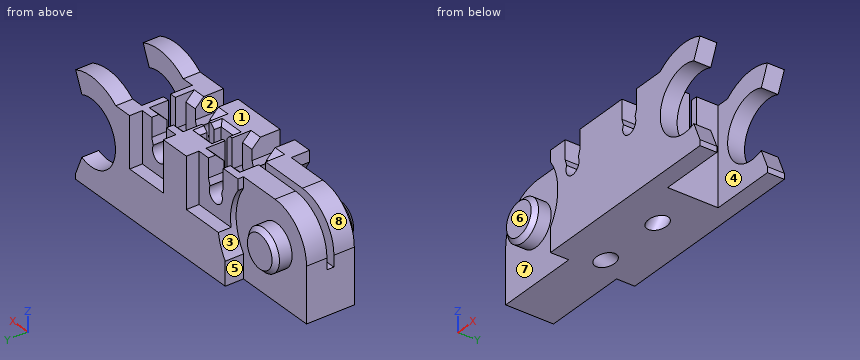
```python
from build123d import *

# Parameters (mm, degrees)
BOSS_EXTRUDE7_DEPTH      = 20
SKETCH2_R                = 4.9175
BOSS_EXTRUDE2_DEPTH      = 4
CUT_EXTRUDE1_REACH       = 70.602
SKETCH3_R                = 7.665
SKETCH4_W                = 4
SKETCH4_H                = 5
CUT_EXTRUDE2_DEPTH       = 10
BOSS_EXTRUDE4_DEPTH      = 4
BOSS_EXTRUDE5_START      = -4
BOSS_EXTRUDE5_DEPTH      = 4
SKETCH25_R               = 12.83
SKETCH25_R_2             = 4.9175
CUT_EXTRUDE9_DEPTH       = 4.33
CUT_EXTRUDE10_START      = -4.33
CUT_EXTRUDE10_DEPTH      = 4.33
CUT_EXTRUDE5_DEPTH       = 70.42587576
SKETCH17_W               = 10.66
SKETCH17_H               = 6.66
CUT_EXTRUDE6_DEPTH       = 7
SKETCH18_W               = 3.2475
SKETCH18_H               = 6.66
SKETCH19_W               = 3.2475
SKETCH19_H               = 6.66
SKETCH20_W               = 51.84
SKETCH20_H               = 1.66
CUT_EXTRUDE7_DEPTH       = 12.66
CHAMFER2_SIZE            = 1
CHAMFER3_SIZE            = 1
CHAMFER4_SIZE            = 2
FILLET1_R                = 10
BOSS_EXTRUDE13_REACH     = 70.3
SKETCH23_W               = 10.34
SKETCH23_H               = 1.66
BOSS_EXTRUDE14_DEPTH     = 0.360269713
SKETCH24_W               = 12.33
SKETCH24_H               = 12
SKETCH24_W_2             = 10.66
CUT_EXTRUDE8_DEPTH       = 3
CHAMFER5_SIZE            = 1
CUT_EXTRUDE11_DEPTH      = 14
CUT_EXTRUDE11_DEPTH_BACK = 14
SKETCH27_R               = 2.0825
SKETCH28_R               = 2.0825
CUT_EXTRUDE12_DEPTH      = 14


with BuildPart() as part:
    # Sketch16 → Boss-Extrude7 (new body)
    with BuildSketch(Plane.XY):
        Polygon((-42.5, -10), (0, -10), (3, -10), (3, -6), (0, -6), (-10.66, -6), (-10.66, 6), (0, 6), (3, 6), (3, 10), (0, 10), (-42.5, 10), (-42.5, 5.67), (-53, 5.67), (-62.5, 5.67), (-62.5, -5.67), (-53, -5.67), (-42.5, -5.67), align=None)
    extrude(amount=BOSS_EXTRUDE7_DEPTH)

    # Sketch2 → Boss-Extrude2 (add)
    with BuildSketch(Plane.XZ.offset(5.67)):
        with Locations(Location((-53, 10, 0), (0, 0, 180))):
            Circle(SKETCH2_R)
    boss_extrude2 = extrude(amount=BOSS_EXTRUDE2_DEPTH)

    # Cut-Extrude1: up to this face of the body (flat: up to its plane)
    cut_extrude1_end = Plane(part.part.faces().sort_by_distance((-19.75, 10, 10))[0])
    # Sketch3 → Cut-Extrude1 (cut, up to the picked face)
    with BuildSketch(Plane.XZ.offset(10), mode=Mode.PRIVATE) as cut_extrude1_sk1:
        with Locations((0, 10)):
            Circle(SKETCH3_R)
    cut_extrude1_tool1 = split(extrude(cut_extrude1_sk1.sketch, amount=-CUT_EXTRUDE1_REACH, mode=Mode.PRIVATE), bisect_by=cut_extrude1_end, keep=Keep.BOTH, mode=Mode.PRIVATE)
    add(cut_extrude1_tool1.solids().sort_by(Axis((0, -10, 10), (0, 1, 0)))[0], mode=Mode.SUBTRACT)

    # Mirror1: Boss-Extrude2 across plane
    add(boss_extrude2.mirror(Plane.ZX))

    # Sketch4 → Cut-Extrude2 (cut)
    with BuildSketch(Plane.XY.offset(20)):
        with Locations((-26.5, 0)):
            Rectangle(SKETCH4_W, SKETCH4_H)
    extrude(amount=-CUT_EXTRUDE2_DEPTH, mode=Mode.SUBTRACT)

    # Sketch10 → Boss-Extrude4 (add)
    with BuildSketch(Plane.XZ.offset(10)):
        with BuildLine():
            Line((3, 17.053525714), (4.956947162, 21.654651425))
            ThreePointArc((4.956947162, 21.654651425), (-12.665, 10), (4.956947162, -1.654651425))
            Line((4.956947162, -1.654651425), (3, 2.946474286))
            ThreePointArc((3, 2.946474286), (-7.665, 10), (3, 17.053525714))
        make_face()
    extrude(amount=-BOSS_EXTRUDE4_DEPTH)

    # Sketch11 → Boss-Extrude5 (add)
    with BuildSketch(Plane(origin=(0, 10, 0), x_dir=(1, 0, 0), z_dir=(0, 1, 0)).offset(BOSS_EXTRUDE5_START)):
        with BuildLine():
            Line((4.956947162, -21.654651425), (3, -17.053525714))
            ThreePointArc((3, -17.053525714), (-7.665, -10), (3, -2.946474286))
            Line((3, -2.946474286), (4.956947162, 1.654651425))
            ThreePointArc((4.956947162, 1.654651425), (-1.632617278, 2.559330628), (-7.771886837, 0))
            Line((-7.771886837, 0), (-10.66, 0))
            Line((-10.66, 0), (-10.66, -20))
            Line((-10.66, -20), (-7.771886837, -20))
            ThreePointArc((-7.771886837, -20), (-1.632617278, -22.559330628), (4.956947162, -21.654651425))
        make_face()
    extrude(amount=BOSS_EXTRUDE5_DEPTH)

    # Sketch25 → Cut-Extrude9 (cut)
    with BuildSketch(Plane.XZ.offset(10)):
        with Locations((-53, 10)):
            Circle(SKETCH25_R)
        with Locations(Location((-53, 10, 0), (0, 0, 180))):
            Circle(SKETCH25_R_2, mode=Mode.SUBTRACT)
    extrude(amount=-CUT_EXTRUDE9_DEPTH, mode=Mode.SUBTRACT)

    # Sketch26 → Cut-Extrude10 (cut)
    with BuildSketch(Plane(origin=(0, 10, 0), x_dir=(1, 0, 0), z_dir=(0, 1, 0)).offset(CUT_EXTRUDE10_START)):
        with BuildLine():
            Line((-42.5, -2.627151161), (-42.5, -17.372848839))
            ThreePointArc((-42.5, -17.372848839), (-40.17, -10), (-42.5, -2.627151161))
        make_face()
    extrude(amount=CUT_EXTRUDE10_DEPTH, mode=Mode.SUBTRACT)

    # Sketch13 → Cut-Extrude5 (cut, through all)
    with BuildSketch(Plane.XZ.offset(10)):
        with BuildLine():
            Line((-37.83, 15.484673169), (-37.83, 20))
            Line((-37.83, 20), (-33.17, 20))
            Line((-33.17, 20), (-33.17, 15.484673169))
            Line((-33.17, 15.484673169), (-33.665, 13.984673169))
            ThreePointArc((-33.665, 13.984673169), (-35.5, 10.9175), (-37.335, 13.984673169))
            Line((-37.335, 13.984673169), (-37.83, 15.484673169))
        make_face()
        with BuildLine():
            Line((-19.83, 15.484673169), (-19.83, 20))
            Line((-19.83, 20), (-15.17, 20))
            Line((-15.17, 20), (-15.17, 15.484673169))
            Line((-15.17, 15.484673169), (-15.665, 13.984673169))
            ThreePointArc((-15.665, 13.984673169), (-17.5, 10.9175), (-19.335, 13.984673169))
            Line((-19.335, 13.984673169), (-19.83, 15.484673169))
        make_face()
    extrude(amount=-CUT_EXTRUDE5_DEPTH, mode=Mode.SUBTRACT)

    # Sketch17 → Cut-Extrude6 (cut)
    with BuildSketch(Plane.XY.offset(20)):
        with Locations((-35.5, 0)):
            Rectangle(SKETCH17_W, SKETCH17_H)
        with Locations((-17.5, 0)):
            Rectangle(SKETCH17_W, SKETCH17_H)
    extrude(amount=-CUT_EXTRUDE6_DEPTH, mode=Mode.SUBTRACT)

    # Sketch18 → Cut-Revolve1 (revolve, cut)
    with BuildSketch(Plane.XY.offset(13)):
        with Locations((-39.20625, 0)):
            Rectangle(SKETCH18_W, SKETCH18_H)
    revolve(axis=Axis((-35.5, 10, 13), (0, -1, 0)), mode=Mode.SUBTRACT)

    # Sketch19 → Cut-Revolve2 (revolve, cut)
    with BuildSketch(Plane.XY.offset(13)):
        with Locations((-21.20625, 0)):
            Rectangle(SKETCH19_W, SKETCH19_H)
    revolve(axis=Axis((-17.5, 10, 13), (0, -1, 0)), mode=Mode.SUBTRACT)

    # Sketch20 → Cut-Extrude7 (cut)
    with BuildSketch(Plane.XY.offset(20)):
        with Locations((-36.58, 0)):
            Rectangle(SKETCH20_W, SKETCH20_H)
    extrude(amount=-CUT_EXTRUDE7_DEPTH, mode=Mode.SUBTRACT)

    # Chamfer2
    chamfer2_edges = [part.edges().sort_by_distance(p)[0] for p in [
        (-48.0825, -9.67, 10),
    ]]
    chamfer(chamfer2_edges, length=CHAMFER2_SIZE)

    # Chamfer3
    chamfer3_edges = [part.edges().sort_by_distance(p)[0] for p in [
        (-48.0825, 9.67, 10),
    ]]
    chamfer(chamfer3_edges, length=CHAMFER3_SIZE)

    # Chamfer4
    chamfer4_edges = [part.edges().sort_by_distance(p)[0] for p in [
        (-31.67, -3.33, 20),
        (-31.67, 3.33, 20),
        (-39.33, 3.33, 20),
        (-39.33, -3.33, 20),
        (-13.67, -3.33, 20),
        (-13.67, 3.33, 20),
        (-21.33, 3.33, 20),
        (-21.33, -3.33, 20),
    ]]
    chamfer(chamfer4_edges, length=CHAMFER4_SIZE)

    # Fillet1
    # the kernel refuses this fillet: 10 mm, written as the material it takes off along each edge
    with BuildSketch(Plane(origin=(-62.5, 30.67, 0), x_dir=(1, 0, 0), z_dir=(0, -1, 0))) as fillet1_piece_1:
        with BuildLine():
            CenterArc((FILLET1_R, FILLET1_R), FILLET1_R, 180, 90)
            Line((0, FILLET1_R), (0, 0))
            Line((0, 0), (FILLET1_R, 0))
        make_face()
    extrude(amount=61.34, mode=Mode.SUBTRACT)
    with BuildSketch(Plane(origin=(-62.5, 30.67, 20), x_dir=(1, 0, 0), z_dir=(0, -1, 0)), Plane(origin=(-62.5, 24.17, 20), x_dir=(1, 0, 0), z_dir=(0, -1, 0))) as fillet1_piece_2:
        with BuildLine():
            CenterArc((FILLET1_R, -FILLET1_R), FILLET1_R, 90, 90)
            Line((0, -FILLET1_R), (0, 0))
            Line((0, 0), (FILLET1_R, 0))
        make_face()
    extrude(amount=54.84, mode=Mode.SUBTRACT)

    # Sketch22 → Boss-Extrude13 (add, up to next)
    with BuildSketch(Plane(origin=(0, 0, -3), x_dir=(-1, 0, 0), z_dir=(0, 0, -1)), mode=Mode.PRIVATE) as boss_extrude13_sk1:
        Polygon((62.5, 5.67), (52.5, 5.67), (42.5, 5.67), (42.5, 10), (7.771886837, 10), (-4.956947162, 10), (-4.956947162, 6), (7.771886837, 6), (10.66, 6), (10.66, -6), (7.771886837, -6), (-4.956947162, -6), (-4.956947162, -10), (7.771886837, -10), (42.5, -10), (42.5, -5.67), (52.5, -5.67), (62.5, -5.67), (62.5, -0.83), (62.139730287, -0.83), (62.139730287, 0.83), (62.5, 0.83), align=None)
    boss_extrude13_tool1 = extrude(boss_extrude13_sk1.sketch, amount=-BOSS_EXTRUDE13_REACH, mode=Mode.PRIVATE) - part.part
    add(boss_extrude13_tool1.solids().sort_by_distance((-29.508071, 0, -3))[0])

    # Sketch23 → Boss-Extrude14 (add)
    with BuildSketch(Plane.ZY.offset(62.139730287)):
        with Locations((2.17, 0)):
            Rectangle(SKETCH23_W, SKETCH23_H)
    extrude(amount=BOSS_EXTRUDE14_DEPTH)

    # Sketch24 → Cut-Extrude8 (cut)
    with BuildSketch(Plane(origin=(0, 10, 0), x_dir=(1, 0, 0), z_dir=(0, 1, 0))):
        with Locations((-36.335, -14)):
            Rectangle(SKETCH24_W, SKETCH24_H)
        with Locations((-17.5, -14)):
            Rectangle(SKETCH24_W_2, SKETCH24_H)
    extrude(amount=-CUT_EXTRUDE8_DEPTH, mode=Mode.SUBTRACT)

    # Chamfer5
    chamfer5_edges = [part.edges().sort_by_distance(p)[0] for p in [
        (-24.5, 1.665, 20),
        (-28.5, -1.665, 20),
        (-26.5, -2.5, 20),
        (-24.5, -1.665, 20),
        (-26.5, 2.5, 20),
        (-28.5, 1.665, 20),
    ]]
    chamfer(chamfer5_edges, length=CHAMFER5_SIZE)

    # Sketch27 → Cut-Extrude11 (cut, two sides: drawn at the far end of the back side and taken through both)
    with BuildSketch(Plane(origin=(-16.214466094, 0, 16.214466094), x_dir=(0, 1, 0), z_dir=(0.7071067811865389, 0, -0.7071067811865561)).offset(-CUT_EXTRUDE11_DEPTH_BACK)):
        with Locations(Location((0, -29.255858544, 0), (0, 0, 270))):
            Circle(SKETCH27_R)
    extrude(amount=CUT_EXTRUDE11_DEPTH + CUT_EXTRUDE11_DEPTH_BACK, mode=Mode.SUBTRACT)

    # Sketch28 → Cut-Extrude12 (cut)
    with BuildSketch(Plane(origin=(-13.901067812, 0, -13.901067812), x_dir=(0, -1, 0), z_dir=(-0.7071067811865389, 0, -0.7071067811865561))):
        with Locations(Location((0, 13.333937944, 0), (0, 0, 90))):
            Circle(SKETCH28_R)
    extrude(amount=-CUT_EXTRUDE12_DEPTH, mode=Mode.SUBTRACT)


solid = part.part
```
Here's how the part is built. I have some questions about the finished solid (model axes, mm). Face numbers are marked on the shaded views. A direction names the side the tool comes from. Give positions to 0.01 mm unless a question says otherwise; leave off trailing zeros. Loops run counter-clockwise (first coordinate to the right, second up) from the corner with the lowest first, then second, coordinate; pieces in that order, holes last. Notation, with made-up numbers: M 63.25,-9.75 L 74.25,-9.75 A12 cw 74.25,-5.75 Z; hole C -2.5,73 d8. An arc over 180 degrees is marked long. Use one line per item in the form item = value. Start each with the question number.
Q1. If we section it at A-A (y = 7.75): Write out the boundary of the cut face in (x, z) (1 decimal).
Q2. If we section it at B-B (x = 0): Write out the boundary of the cut face in (y, z) (3 decimals).
Q3. Thinking about a two-plate mould opening in X: for the marked faces 6, 7 and 8, which applies, +X half, -X half, draft (parallel to the pull), parting line (faces both ways), or undercut?
Q4. If we section it at D-D (x = -7): Write out the boundary of the cut face in (y, z), then the cut area to 3 significant figures.
Q5. I need wall thicknesses on line 1 along Y through (x, z) = (-13, 10.5); line 2 along X through (y, z) = (8.75, 10) (1 decimal); line 3 along Y through (x, z) = (-45, 13.75). Which ranges of each line are inside material? Lowest first, please.
Q6. Will these pins go through, and if not, where does the flat tip stop? pin 1 Ø5 at (y, z) = (2.5, 16.5) entering from +X; pin 2 Ø4 at (y, z) = (4.5, 18.5) entering from -X; pin 3 Ø6 at (x, y) = (-10, -7) entering from +Z.
Q7. Which directions (+Z, -Z, +X, -X, +Y, -Y) give clear straight access to the entire face, cutting with the end or side of a thin tool? Please do the marked faces 1, 2, 3, 4 and 5.
Q8. If we section it at C-C (z = 12.25): State how many separate pieces and enclosed holes the cut face has, then the cut area to 3 significant figures.
Taken from the geometry:
q1.outline = C -53,10 d9.8; M -42.5,-3 L 5,-3 L 5,-1.7 L 3,2.9 A7.7 cw long 3,17.1 L 5,21.7 A12.7 ccw -7.8,20 L -12.2,20 L -12.2,8 L -22.8,8 L -22.8,20 L -30.2,20 L -30.2,8 L -40.3,8 A12.8 cw -42.5,2.6 Z
q2.outline = M -10,-3 L -6,-3 L -6,2.335 L -10,2.335 Z; M -10,17.665 L -6,17.665 L -6,22.665 L -10,22.665 Z; M 6,-3 L 10,-3 L 10,2.335 L 6,2.335 Z; M 6,17.665 L 10,17.665 L 10,22.665 L 6,22.665 Z
q3.face_6 = draft
q3.face_7 = undercut
q3.face_8 = -X half
q4.outline = M -10,-3 L -6,-3 L -6,6.88 L -10,6.88 Z; M -10,13.12 L -6,13.12 L -6,20.55 L -10,20.55 Z; M 6,-3 L 10,-3 L 10,6.88 L 6,6.88 Z; M 6,13.12 L 10,13.12 L 10,20.55 L 6,20.55 Z
q4.area = 138 mm^2
q5.line_1 = -10 to -3.33, 3.33 to 7
q5.line_2 = -57.8 to -48.2, -30.2 to -22.8, -12.2 to -7.7
q5.line_3 = -5.67 to -0.83, 0.83 to 5.67
q6.pin_1 = -10.66
q6.pin_2 = -60.1
q6.pin_3 = 20.55
q7.face_1 = +Z, -X, +Y, -Y
q7.face_2 = +Z, +Y, -Y
q7.face_3 = +Y
q7.face_4 = +Z, -Z, +X
q7.face_5 = +Z, -Z, -X, +Y
q8.separate_pieces = 6
q8.enclosed_holes = 0
q8.area = 589 mm^2
